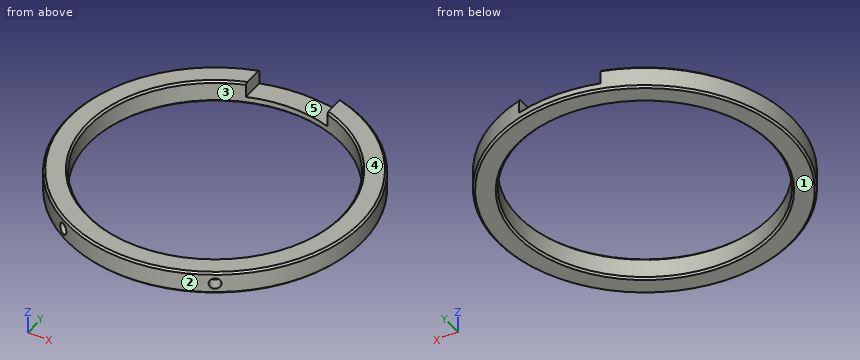
Autodesk Inventor part; units mm, degrees
ref_plane "工作平面1" through (0, 0, 3) normal (0, 0, 1) x (1, 0, 0)
ref_plane "工作平面2" through (20.55, -34.201, 3) normal (0.515, -0.8572, 0) x (0.8572, 0.515, 0)
ref_plane "工作平面3" through (-20.55, -34.201, 3) normal (-0.515, -0.8572, 0) x (0.8572, -0.515, 0)
sketch "草圖1" plane through (0, 0, 0) normal (0, 0, 1) x (1, 0, 0)
  circle A0 centre (0, 0) radius 39.9
  circle A1 centre (0, 0) radius 34.1
  dimension "d0" = 79.8
  dimension "d3" = 68.2
extrude "擠出1" add sketch "草圖1" along normal blind 6
sketch "草圖2" plane through (0, 0, 6) normal (0, 0, 1) x (1, 0, 0)
  circle A0 centre (0, 0) radius 34.1
  circle A1 centre (0, 0) radius 39.9
  line L0 (0, 0) -> (0, 39.9)
  line L1 (11, 40.6521) -> (11, 12.8237)
  line L2 (-11, 40.6521) -> (-11, 12.8237)
  line L3 (-11, 40.6521) -> (11, 40.6521)
  line L4 (-11, 12.8237) -> (11, 12.8237)
  point P0 (11, 38.3537)
  point P1 (11, 32.2771)
  point P2 (-11, 38.3537)
  point P3 (-11, 32.2771)
  dimension "d6" = 22
extrude "擠出2" cut sketch "草圖2" against normal blind 4 contours A0 L0 A1 L1 | L2 A1 L0 A0
ref_plane "工作平面1" through (0, 0, 3) normal (0, 0, 1) x (1, 0, 0)
sketch "草圖3" plane through (0, 0, 3) normal (0, 0, 1) x (1, 0, 0)
  line L0 (0, 0) -> (0, -42.4806)
  line L1 (0, 0) -> (-20.55, -34.201)
  line L2 (0, 0) -> (20.55, -34.201)
  arc A0 (-11, 38.3537) -> (11, 38.3537) centre (0, 0) ccw
  line L3 (-20.55, -34.201) -> (20.55, -34.201)
  dimension "d27" = 31
ref_plane "工作平面2" through (20.55, -34.201, 3) normal (0.515, -0.8572, 0) x (0.8572, 0.515, 0)
ref_plane "工作平面3" through (-20.55, -34.201, 3) normal (-0.515, -0.8572, 0) x (0.8572, -0.515, 0)
sketch "草圖4" plane through (20.55, -34.201, 3) normal (0.515, -0.8572, 0) x (0.8572, 0.515, 0)
  point P0 (0, -3)
  point P1 (0, 0)
hole "孔1" at (20.55, -34.201, 3) direction (-0.515, 0.8572, 0) diameter 3 depth 3.5 tip angle 118
sketch "草圖5" plane through (-20.55, -34.201, 3) normal (-0.515, -0.8572, 0) x (0.8572, -0.515, 0)
  point P0 (0, -3)
  point P1 (0, 0)
hole "孔2" at (-20.55, -34.201, 3) direction (0.515, 0.8572, 0) diameter 3 depth 3.5 tip angle 118
chamfer "倒角1" distance 0.5 angle 45 6 edges at (-19.8458, -27.73, 6) (27.73, 19.8458, 6) (-34.1, 0, 0) (-24.0116, -31.8662, 6) (31.8662, 24.0116, 6) (-39.9, 0, 0)
properties part number "KE-SP-02-P1"
Check sheet for the modelled part. Datum: model origin and axes. Units: mm. Face numbers are marked on the shaded views. A direction names the side the tool comes from. Round coordinates to 2 decimals unless told otherwise and drop trailing zeros. Order: outer loops, then holes, each group sorted by start corner. A loop starts at its lowest first (then second) coordinate and runs counter-clockwise, first axis right, second up. Notation, with made-up numbers: M 74.25,68.25 L 93.25,68.25 A12 cw 93.25,72.25 Z; hole C -31,6 d11. An arc over 180 degrees is marked long. One line per item, written item: value. Start each with the question number.
1. Release check for a two-part mould opening along Y. For the marked faces 1, 2 and 3 record: released by +Y, released by -Y, zero draft, split by the parting line, or undercut.
2. Gauge pin test, flat ends, axial feed: P1, Ø3, axis at y = 2, z = 3, coming from the +X side; P2, Ø1.2, axis at y = 34.5, z = 4.5, coming from the +X side; P3, Ø8.5, axis at x = 0.5, y = 36, coming from the +Z side. Record the tip position at first contact, or that the pin passes through.
3. Section check A-A on x = 0. Enter the section's corners in (y, z), and give its area (4 significant figures).
4. Scan lines: line 1 along X through (y, z) = (34.5, 3.5); line 2 along X through (y, z) = (0, 3.05); line 3 along Y through (x, z) = (0, 2.05). Record each from-to range of solid material in increasing order.
5. Access from +Z, -Z, +X, -X, +Y, -Y to the whole of each face (thin tool, end or side, straight path). Record for the marked faces 4 and 5.
6. Section check B-B on y = 0. Enter the section's corners in (x, z).
Results found:
1. face 1: zero draft
1. face 2: split by the parting line
1. face 3: undercut
2. P1: x = 39.9
2. P2: x = 21.04
2. P3: z = 2
3. outline: M -39.9,0.5 L -39.4,0 L -34.6,0 L -34.1,0.5 L -34.1,5.5 L -34.6,6 L -39.4,6 L -39.9,5.5 Z; M 34.1,0.5 L 34.6,0 L 39.4,0 L 39.9,0.5 L 39.9,2 L 34.1,2 Z
3. area: 45.65 mm^2
4. line 1: -20.04 to -11, 11 to 20.04
4. line 2: -39.9 to -34.1, 34.1 to 39.9
4. line 3: -39.9 to -34.1
5. face 4: +Z, +X, -X, +Y, -Y
5. face 5: +Z, +Y
6. outline: M -39.9,0.5 L -39.4,0 L -34.6,0 L -34.1,0.5 L -34.1,5.5 L -34.6,6 L -39.4,6 L -39.9,5.5 Z; M 34.1,0.5 L 34.6,0 L 39.4,0 L 39.9,0.5 L 39.9,5.5 L 39.4,6 L 34.6,6 L 34.1,5.5 Z
